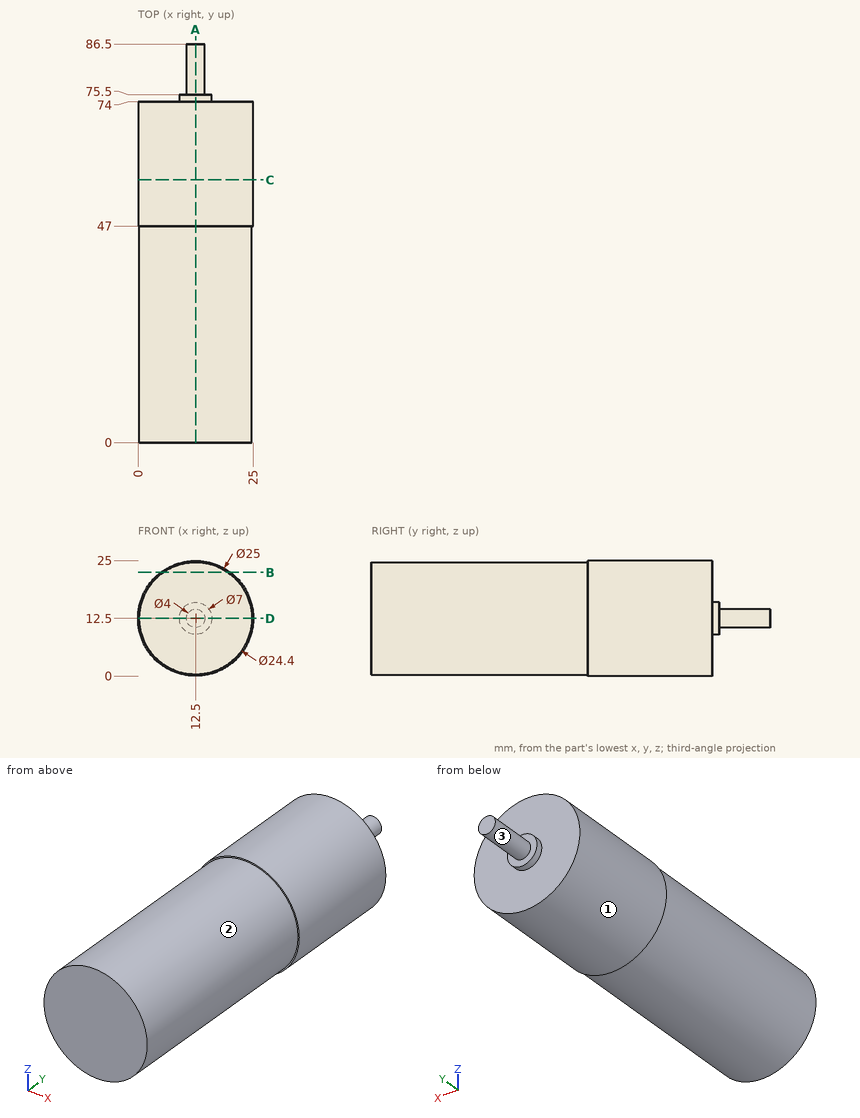
Answer from the drawing. Dimensions are ordinates in mm from the lowest x, y and z of the part. A direction names the side the tool comes from. Coordinates: 2 decimals unless noted, no trailing zeros. Order: outer loops, then holes, each group sorted by start corner. A loop starts at its lowest first (then second) coordinate and runs counter-clockwise, first axis right, second up. Notation, with made-up numbers: (73.5, -1) - (107.5, -1) arc R22 cw to (107.5, 30) - close; hole circle Ø10 at (81, 51.25). An arc over 180 degrees is marked (long way). Put each result on its own line as item: value. Start each with the question number.
1) Find section B-B (z = 22.5). Give the vertices of the cut face in (x, y).
2) For the marked faces 1, 2 and 3, determine the directions among +Z, -Z, +X, -X, +Y, -Y from which every point of the face is accessible in a straight line to the end or side of a thin tool.
3) Flat-ended cylindrical pins translate along their axes: pin 1 (4 mm diameter, centred on x = 5, z = 2.5, fed in from +Y); pin 2 (6 mm diameter, centred on x = 12.5, z = 15.5, fed in from -Y); pin 3 (4 mm diameter, centred on y = 31.5, z = 3, fed in from -X); pin 4 (6 mm diameter, centred on y = 15, z = 18.5, fed in from +X). Find the tip coordinate at first contact, or state that the pin passes through.
4) Find the intervals of material crossed by line 1 (X direction, y = 38.5, z = 12); line 2 (Y direction, x = 19.25, z = 4.25); line 3 (X direction, y = 49.5, z = 12.25), in increasing order. Write a range as from..to.
5) Find section A-A (x = 12.5). Give the vertices of the cut face in (y, z), plus the area to 3 significant figures.
6) Find section C-C (y = 57). Give the vertices of the cut face in (x, z), plus the area to 3 significant figures.
7) Find section D-D (z = 12.5). Give the vertices of the cut face in (x, y), plus the area to 3 significant figures.
Results list:
1. outline: (5, 47) - (5.51, 47) - (5.51, 0) - (19.49, 0) - (19.49, 47) - (20, 47) - (20, 74) - (5, 74) - close
2. face 1: +Y, -Y
2. face 2: -Y
2. face 3: +Y
3. pin 1: stops at y = 74
3. pin 2: stops at y = 0
3. pin 3: stops at x = 2.88
3. pin 4: stops at x = 24.33
4. line 1: x = 0.31..24.69
4. line 2: y = 0..74
4. line 3: x = 0..25
5. outline: (0, 0.3) - (47, 0.3) - (47, 0) - (74, 0) - (74, 9) - (75.5, 9) - (75.5, 10.5) - (86.5, 10.5) - (86.5, 14.5) - (75.5, 14.5) - (75.5, 16) - (74, 16) - (74, 25) - (47, 25) - (47, 24.7) - (0, 24.7) - close
5. area: 1,880 mm^2
6. outline: circle Ø25 at (12.5, 12.5)
6. area: 491 mm^2
7. outline: (0, 47) - (0.3, 47) - (0.3, 0) - (24.7, 0) - (24.7, 47) - (25, 47) - (25, 74) - (16, 74) - (16, 75.5) - (14.5, 75.5) - (14.5, 86.5) - (10.5, 86.5) - (10.5, 75.5) - (9, 75.5) - (9, 74) - (0, 74) - close
7. area: 1,880 mm^2
